from build123d import *

# Parameters (mm, degrees)
EXTRUDE1_DEPTH     = 40
CUT_EXTRUDE3_DEPTH = 2.42


with BuildPart() as part:
    # Sketch1 → Extrude1 (new body)
    with BuildSketch(Plane.XY):
        Polygon((0, 0), (0, -25.22), (25.22, -25.22), (25.22, -23.8), (1.42, -23.8), (1.42, 0), align=None)
    extrude(amount=EXTRUDE1_DEPTH)

    # Sketch3 → Cut-Extrude3 (cut, through all)
    with BuildSketch(Plane(origin=(0, -23.8, 0), x_dir=(-1, 0, 0), z_dir=(0, 1, 0))):
        Polygon((-25.22, 0), (-25.22, 20.6), (-17.85, 20.6), (-17.85, 18), (-10.8, 18), (-10.8, 20.6), (-2.84, 20.6), (-2.84, 23.5), (-1.42, 23.5), (-1.42, 0), align=None)
    extrude(amount=-CUT_EXTRUDE3_DEPTH, mode=Mode.SUBTRACT)


solid = part.part
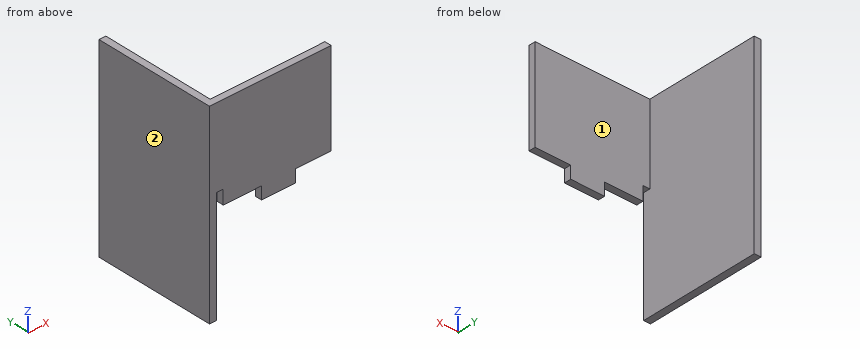
The model under review builds one solid part; all positions refer to its coordinate system, in mm. Face numbers are marked on the shaded views. A direction names the side the tool comes from. Round coordinates to 2 decimals unless told otherwise and drop trailing zeros. Write each loop counter-clockwise with the first axis right and the second up, starting at its lowest first coordinate (ties: lowest second). Pieces come first, ordered by that corner, then holes. Notation, with made-up numbers: (67.5, 46) - (99.5, 46) arc R21 cw to (99.5, 83) - close; hole circle Ø6 at (-22, 30.5). An arc over 180 degrees is marked (long way). One line per item, written item: value. Start each with the question number.
1. Consider section D-D on x = 19. Write out the cut boundary in (y, z).
2. Clearance check with flat-ended pins moving along their axes: P1, Ø5, axis at y = -4.5, z = 33.5, coming from the +X side; P2, Ø1.1, axis at x = 21.5, y = -25, coming from the -Z side; P3, Ø11, axis at x = 8, z = 33, coming from the +Y side; P4, Ø1.6, axis at x = 2, y = -24.5, coming from the -Z side. State where each tip first meets the part, or that it passes through.
3. To check wall thickness, follow L1, parallel to X at y = -5.75, z = 34; L2, parallel to Y at x = 17.5, z = 28. State the ranges of each line that lie inside material, in increasing order. Write a range as from..to.
4. Consider section A-A on z = 18.5. Write out the cut boundary in (x, y), and give its area (3 significant figures).
5. Machinability: for the marked faces 1 and 2, which of the approach directions +Z, -Z, +X, -X, +Y, -Y give a long, thin tool a straight path to every point of the face, cutting with its end or side? Answer none if there is none.
6. Consider section B-B on z = 35. Write out the cut boundary in (x, y).
7. Consider section C-C on y = -12. Write out the cut boundary in (x, z), and give its area (3 significant figures).
Checks:
1. outline: (-25.22, 20.6) - (-23.8, 20.6) - (-23.8, 40) - (-25.22, 40) - close
2. P1: stops at x = 1.42
2. P2: stops at z = 20.6
2. P3: stops at y = -23.8
2. P4: stops at z = 0
3. L1: x = 0..1.42
3. L2: y = -25.22..-23.8
4. outline: (0, -25.22) - (1.42, -25.22) - (1.42, 0) - (0, 0) - close; (10.8, -25.22) - (17.85, -25.22) - (17.85, -23.8) - (10.8, -23.8) - close
4. area: 45.8 mm^2
5. face 1: +Z, -Z, +X, +Y
5. face 2: +Z, -Z, -X, +Y, -Y
6. outline: (0, -25.22) - (25.22, -25.22) - (25.22, -23.8) - (1.42, -23.8) - (1.42, 0) - (0, 0) - close
7. outline: (0, 0) - (1.42, 0) - (1.42, 40) - (0, 40) - close
7. area: 56.8 mm^2
